Answer from the drawing. Dimensions are ordinates in mm from the lowest x, y and z of the part. A direction names the side the tool comes from. Coordinates: 2 decimals unless noted, no trailing zeros. Write each loop counter-clockwise with the first axis right and the second up, starting at its lowest first coordinate (ties: lowest second). Pieces come first, ordered by that corner, then holes.
(1) Which of the six approach directions +Z, -Z, +X, -X, +Y, -Y give full straight-line access (tool end or side, diameter ignored) to the marked faces 4 and 5?
(2) For a pull along Y with two mould halves and no side action, classify the marked faces 1, 2 and 3 as +Y half, -Y half, draft (parallel to the pull), parting line (faces both ways), or undercut.
(3) The part is cut by section D-D on x = 9.5. Determine the outline of the cut face in (y, z).
(4) The part is cut by section C-C on z = 3.75. Determine the outline of the cut face in (x, y) (1 decimal).
(5) The part is cut by section A-A on x = 5. Determine the outline of the cut face in (y, z).
(6) Given P1, Ø8, axis at y = 5.5, z = 6, coming from the -X side; P2, Ø7, axis at x = 5, z = 3.5, coming from the -Y side; P3, Ø3, axis at y = 9, z = 10.5, coming from the -X side; P4, Ø1.5, axis at x = 9.5, y = 10.5, coming from the +Z side, each flat-ended and moving along its own axis, determine where each tip first touches the part or whether it passes through.
(7) Straight lines are drawn through the part: line 1 (Y direction, x = 4.75, z = 10.25); line 2 (X direction, y = 8.75, z = 4); line 3 (Z direction, x = 9, y = 4) (1 decimal). For each, find the intervals that lie inside material, in ascending order.
(8) The part is cut by section B-B on y = 13. Determine the outline of the cut face in (x, z) (1 decimal).
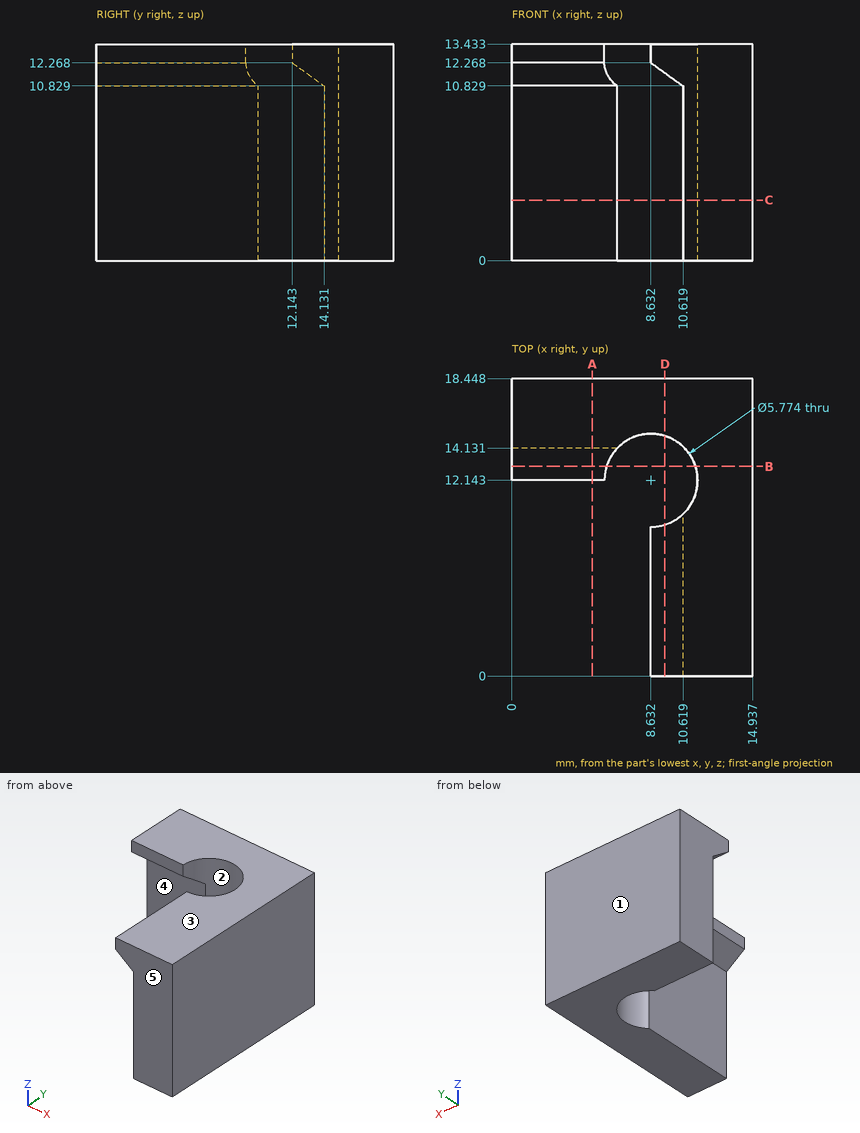
Model answer:
1. face 4: -Z, -X, -Y
1. face 5: +Z, -Z, +X, -X, -Y
2. face 1: +Y half
2. face 2: undercut
2. face 3: draft
3. outline: (0, 11.64) - (9.39, 11.64) - (9.39, 13.43) - (0, 13.43) - close; (14.9, 0) - (18.45, 0) - (18.45, 13.43) - (14.9, 13.43) - close
4. outline: (0, 14.1) - (6.5, 14.1) arc R2.9 cw (long way) to (10.6, 10) - (10.6, 0) - (14.9, 0) - (14.9, 18.4) - (0, 18.4) - close
5. outline: (12.14, 12.27) - (14.13, 10.83) - (14.13, 0) - (18.45, 0) - (18.45, 13.43) - (12.14, 13.43) - close
6. P1: stops at x = 10.62
6. P2: stops at y = 14.13
6. P3: stops at x = 9
6. P4: passes through
7. line 1: y = 14.13 to 18.45
7. line 2: x = 10.62 to 14.94
7. line 3: z = 12 to 13.4
8. outline: (0, 11.6) - (5.9, 11.6) - (5.9, 13.4) - (0, 13.4) - close; (11.4, 0) - (14.9, 0) - (14.9, 13.4) - (11.4, 13.4) - close
